Autodesk Inventor part; units mm, degrees
ref_plane "Work Plane1" through (29, 0, 0) normal (0, -1, 0) x (1, 0, 0)
ref_plane "YZ Plane" through (0, 0, 0) normal (1, 0, 0) x (0, 1, 0)
ref_plane "XZ Plane" through (0, 0, 0) normal (0, 1, 0) x (-1, 0, 0)
sketch "Sketch1" plane through (0, 0, 0) normal (0, 0, 1) x (1, 0, 0)
  line L0 (0.1133, 0) -> (55, 0)
  line L1 (55, 0) -> (55, 3)
  line L2 (55, 3) -> (31, 3)
  line L3 (31, 3) -> (30.3864, 3)
  line L4 (30.3864, 3) -> (0, 3)
  line L5 (0, 3) -> (0, 5.25)
  line L6 (0, 5.25) -> (-3.3, 5.25)
  line L7 (-3.3, 5.25) -> (-3.3, 2.3094)
  line L8 (-3.3, 2.3094) -> (-1.22, 2.3094)
  line L9 (-1.22, 2.3094) -> (0.1133, 0)
  line L10 (-14.96, 0) -> (66.66, 0)
  line L11 (0, -1.05) -> (0, 6.3)
  line L12 (31, 3) -> (0, 3) construction
  dimension "d1" = 24
  dimension "d2" = 0.6136
  dimension "d3" = 3.3
  dimension "d4" = 2.08
  dimension "d5" = 60
  dimension "d6" = 6
  dimension "d7" = 6
  dimension "d8" = 4.6188
  dimension "d9" = 10.5
  dimension "d26" = 55
revolve "Body" add sketch "Sketch1" angle 360 about axis through (0.1133, 0, 0) along (1, 0, 0) contours L9 L11 L4 L3 L2 L1 L0 | L9 L8 L7 L6 L5 L11
sketch "Sketch2" plane through (-3.3, 0, 0) normal (-1, 0, 0) x (0, 0, 1)
  circle A0 centre (0, 0) radius 2.3094
  line L0 (0, -7.35) -> (0, 7.35)
  line L1 (-7.35, 0) -> (7.35, 0)
  line L2 (2.3094, 0) -> (1.1547, -2)
  line L3 (1.1547, -2) -> (-1.1547, -2)
  line L4 (-1.1547, -2) -> (-2.3094, 0)
  line L5 (-2.3094, 0) -> (-1.1547, 2)
  line L6 (-1.1547, 2) -> (1.1547, 2)
  line L7 (1.1547, 2) -> (2.3094, 0)
extrude "Slot" add sketch "Sketch2" against normal up to next contours L7 A0 | A0 L2 | L6 L0 A0 | A0 L0 L3 | L0 L6 A0 | A0 L3 L0 | L4 A0 | A0 L5
fillet "Fillet1" radius 2.56 1 edges at (-3.3, -5.25, 0)
thread "Thread"
chamfer "Chamfer1" distance 0.6135 distance2 0.6135 1 edges at (55, -3, 0) measured on face at (55, 0.1411, 0.823)
ref_plane "Work Plane1" through (29, 0, 0) normal (0, -1, 0) x (1, 0, 0)
fillet "Fillet2" radius 0.25 1 edges at (0, -3, 0)
equation "\"d1\" = GEL"
equation "\"d3\" = KOH"
equation "\"d4\" = INTI"
equation "\"d6\" = GD"
equation "\"d7\" = BDM"
equation "\"d8\" = 1.1547 * SW"
equation "\"d9\" = KOD"
equation "\"d26\" = NLG"
equation "\"d30\" = R"
equation "\"d17\" = RR"
equation "\"d13\" = GEL"
equation "\"d15\" = -0.5 * SPD + 0.5 * GD"
equation "\"d16\" = GUL"
equation "\"GD\" = NND"
equation "\"NLG\" = 55"
equation "\"GEL\" = 24"
equation "\"KOD\" = 10.5"
equation "\"KOH\" = 3.3"
equation "\"INTI\" = 2.08"
equation "\"GAL\" = 0.61345 * PTC"
equation "\"GUL\" = 0.61345 * PTC"
equation "\"BDM\" = NND"
equation "\"SW\" = 4"
equation "\"RR\" = 2.56"
equation "\"SPD\" = NND - 1.2269 * PTC"
equation "\"R\" = 0.25"
equation "\"TOA\" = 30deg"
equation "\"GD1\" = THREADDIA - 1.2269 * PTC"
equation "\"THREADDIA\" = 6"
equation "\"PTC\" = 1"
equation "\"NND\" = 6"
equation "\"KOH1\" = 0.74"
equation "\"E0\" = 4.583"
properties part number "ISO 7380-1 - M6 x 55" material "Steel"
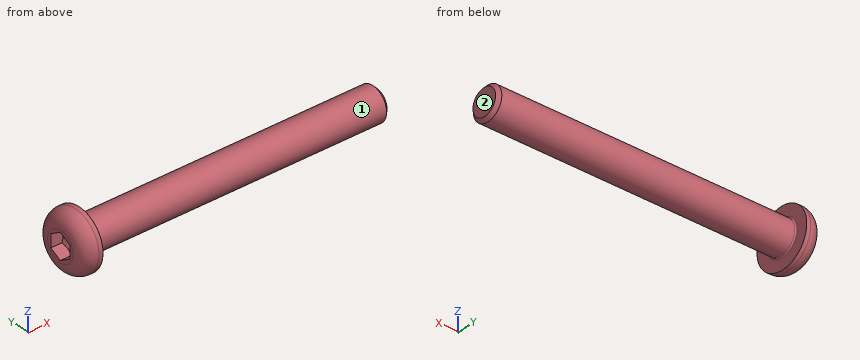
Can you work these out from the model? Positions are in its coordinate system, mm. Face numbers are marked on the shaded views. A direction names the side the tool comes from. Coordinates: 2 decimals unless noted, no trailing zeros. Write each loop counter-clockwise with the first axis right and the second up, starting at its lowest first coordinate (ties: lowest second). Pieces come first, ordered by that corner, then holes. Notation, with made-up numbers: (-10.5, 17.5) -> (44.5, 17.5) arc R24 ccw to (44.5, 44.5) -> close; hole circle Ø7 at (-22, 53). An arc over 180 degrees is marked (long way). Write each question's results on one line, items separated by ' | '. Start each with the question number.
Q1. Imagine slicing it at A-A (x = 10.5). Write out the boundary of the cut face in (y, z).
Q2. On a 3-axis mill with a long thin cutter (end or side, diameter ignored), from which of +Z, -Z, +X, -X, +Y, -Y can I reach the whole of each face in a straight line? I mean the marked faces 1 and 2. Say none if no direction works.
Q3. I'm going to push flat-ended pins straight in: pin 1 (2.5 mm diameter, centred on x = -2.5, z = -0.5, fed in from -Y); pin 2 (0.7 mm diameter, centred on x = -2.5, z = 0, fed in from +Y); pin 3 (2 mm diameter, centred on x = 21, y = -3.5, fed in from -Z); pin 4 (6 mm diameter, centred on y = -3.5, z = -2.5, fed in from -X). Where does each tip first touch, or does it pass through?
Q4. If I drill on probe 1 along Z at (x, y) = (4, -0.25); probe 2 along X at (y, z) = (0, -2); probe 3 along Z at (x, y) = (3.5, 2.5), over which ranges is the centre line in solid material (lowest first)?
Taken from the geometry:
1) outline: circle Ø6 at (0, 0)
2) face 1: +X | face 2: +Z, -Z, +X, +Y, -Y
3) pin 1: stops at y = -5.19 | pin 2: stops at y = 4.83 | pin 3: stops at z = -1.66 | pin 4: stops at x = -3.3
4) probe 1: z = -2.99 to 2.99 | probe 2: x = -1.04 to 55 | probe 3: z = -1.66 to 1.66
